```python
from build123d import *

# Parameters (mm, degrees)
SKETCH1_R           = 2.25
BOSS_EXTRUDE1_DEPTH = 12.7
SKETCH2_W           = 25.4
SKETCH2_H           = 25.4
BOSS_EXTRUDE2_DEPTH = 25.4
SKETCH3_W           = 25.4
SKETCH3_H           = 12.7
CUT_EXTRUDE1_DEPTH  = 25.4
FILLET2_R           = 6.35
FILLET3_R           = 12.7
SKETCH4_R           = 2
CUT_EXTRUDE2_DEPTH  = 25.4


with BuildPart() as part:
    # Sketch1 → Boss-Extrude1 (new body)
    with BuildSketch(Plane.XY):
        with BuildLine():
            Line((19.05, 12.7), (0, 12.7))
            ThreePointArc((0, 12.7), (-12.7, 0), (0, -12.7))
            Line((0, -12.7), (19.05, -12.7))
            Line((19.05, -12.7), (19.05, 12.7))
        make_face()
        Circle(SKETCH1_R, mode=Mode.SUBTRACT)
    extrude(amount=BOSS_EXTRUDE1_DEPTH)

    # Sketch2 → Boss-Extrude2 (add)
    with BuildSketch(Plane(origin=(19.05, 0, 0), x_dir=(0, 0, -1), z_dir=(1, 0, 0))):
        with Locations((-6.35, 0)):
            Rectangle(SKETCH2_W, SKETCH2_H)
    extrude(amount=BOSS_EXTRUDE2_DEPTH)

    # Sketch3 → Cut-Extrude1 (cut)
    with BuildSketch(Plane.XY.offset(19.05)):
        with Locations((31.75, 0)):
            Rectangle(SKETCH3_W, SKETCH3_H)
    extrude(amount=-CUT_EXTRUDE1_DEPTH, mode=Mode.SUBTRACT)

    # Fillet2
    fillet2_edges = [part.edges().sort_by_distance(p)[0] for p in [
        (19.05, 9.525, 19.05),
        (19.05, -9.525, 19.05),
        (19.05, -9.525, -6.35),
        (19.05, 9.525, -6.35),
    ]]
    fillet(fillet2_edges, radius=FILLET2_R - 0.0001)  # a hair under: the kernel refuses the full size

    # Fillet3
    fillet3_edges = [part.edges().sort_by_distance(p)[0] for p in [
        (44.45, 9.525, 19.05),
        (44.45, -9.525, 19.05),
        (44.45, 9.525, -6.35),
        (44.45, -9.525, -6.35),
    ]]
    fillet(fillet3_edges, radius=FILLET3_R - 0.0001)  # a hair under: the kernel refuses the full size

    # Sketch4 → Cut-Extrude2 (cut)
    with BuildSketch(Plane(origin=(0, 12.7, 0), x_dir=(1, 0, 0), z_dir=(0, 1, 0))):
        with Locations(Location((31.75, -6.35, 0), (0, 0, 270))):
            Circle(SKETCH4_R)
    extrude(amount=-CUT_EXTRUDE2_DEPTH, mode=Mode.SUBTRACT)


solid = part.part
```
CAD build for the part. Positions are in the model's coordinates, mm. A direction names the side the tool comes from. Give positions to 0.01 mm unless a question says otherwise; leave off trailing zeros. Order: outer loops, then holes, each group sorted by start corner. A loop starts at its lowest first (then second) coordinate and runs counter-clockwise, first axis right, second up.
(1) Saw through at C-C, the plane z = 10. Give the cut face in (x, y), then the cut area to 3 significant figures.
(2) Drill centre lines: L1, parallel to X at y = -0.25, z = 6; L2, parallel to Y at x = 40, z = 1.75; L3, parallel to X at y = 11, z = 6.35. Where is each one in solid material? Low to high.
(3) Saw through at A-A, the plane y = 0. Give the cut face in (x, z).
(4) Saw through at D-D, the plane x = 17. Give the cut face in (y, z), then the cut area to 3 significant figures.
(5) Tool access for faces 4 (the flat face through (3, 0, 0)), 5 (the flat face through (3, 0, 12.7)), 6 (the flat face through (29, -10, 19.05)): list every direction of +Z, -Z, +X, -X, +Y, -Y with a clear straight run to the whole face (end or side of a thin tool).
(6) Mould opens along Y. For faces 1 (the flat face through (22, -12.7, 7)), 2 (the cylindrical face through (20.86, -9.48, -4.44)), 3 (the flat face through (19.05, 0, 6)) say: released by +Y, released by -Y, zero draft, split by the parting line, or undercut.
(7) Saw through at B-B, the plane x = 28. Give the cut face in (y, z).
(8) Flat gauge pins, fed straight in: pin 1 (8 mm diameter, centred on y = 7, z = 1, fed in from -X); pin 2 (4 mm diameter, centred on y = -0.5, z = 9.5, fed in from +X); pin 3 (5 mm diameter, centred on x = -1.5, y = -7.5, fed in from -Z). Where does each tip first touch, or does it go through?
Results found:
1. outline: (0, -12.7) - (43.91, -12.7) - (43.91, -6.35) - (19.05, -6.35) - (19.05, 6.35) - (43.91, 6.35) - (43.91, 12.7) - (0, 12.7) arc R12.7 ccw to start; hole circle Ø4.5 at (0, 0)
1. area: 1,040 mm2
2. L1: x = -12.7 to -2.24, 2.24 to 19.05
2. L2: y = -12.7 to -6.35, 6.35 to 12.7
2. L3: x = -6.35 to 29.75, 33.75 to 44.45
3. outline: (-12.7, 0) - (-2.25, 0) - (-2.25, 12.7) - (-12.7, 12.7) - close; (2.25, 0) - (19.05, 0) - (19.05, 12.7) - (2.25, 12.7) - close
4. outline: (-12.7, 0) - (12.7, 0) - (12.7, 12.7) - (-12.7, 12.7) - close
4. area: 323 mm2
5. face 4: -Z, -X, +Y, -Y
5. face 5: +Z, -X, +Y, -Y
5. face 6: +Z, +X, -X, +Y, -Y
6. face 1: released by -Y
6. face 2: zero draft
6. face 3: undercut
7. outline: (-12.7, -6.35) - (-6.35, -6.35) - (-6.35, 19.05) - (-12.7, 19.05) - close; (6.35, -6.35) - (12.7, -6.35) - (12.7, 19.05) - (6.35, 19.05) - close
8. pin 1: stops at x = -12.34
8. pin 2: stops at x = 19.05
8. pin 3: stops at z = 0
